Input: part model. Units: mm. Frame: model coordinates. Face numbers are marked on the shaded views. A direction names the side the tool comes from. Coordinates: 2 decimals unless noted, no trailing zeros. Loops run counter-clockwise (first coordinate to the right, second up) from the corner with the lowest first, then second, coordinate; pieces in that order, holes last. Notation, with made-up numbers: (-21, 19.5) - (-2, 19.5) arc R25 cw to (-2, 52.5) - close; hole circle Ø9 at (6.5, 55.25). An arc over 180 degrees is marked (long way). Use a Markdown table: item, result. Add a question column.
1. Section query B-B on z = 3.25. Return the cut outline in (x, y).
2. Draft query along X for the marked faces 4, 5 and 6. Return one class per face: released by +X, released by -X, zero draft, split by the parting line, or undercut.
3. Contact query for flat-ended pins moving along their axis: P1, Ø8, axis at y = -5.5, z = 8, coming from the +X side; P2, Ø1.9, axis at y = 27.5, z = -3.5, coming from the +X side; P3, Ø3.5, axis at y = 29.5, z = 4.5, coming from the -X side. Output: stop coordinate, or through.
4. Section query A-A on z = 7.5. Return the cut outline in (x, y).
5. Ray query, L1, parallel to Y at x = -4.5, z = 9; L2, parallel to X at y = -29, z = 1; L3, parallel to Z at x = 4, y = 5. Return the intervals inside material, ascending. Write a range as [from, to].
6. Section query C-C on y = -16. Return the cut outline in (x, z), then the cut area to 3 significant figures.
7. Section query D-D on x = 9.5. Return the cut outline in (y, z).
8. Access query for the marked faces 1, 2 and 3. Directions: +Z, -Z, +X, -X, +Y, -Y. A direction counts if a zero-diameter tool reaches every point of the face in a straight line with its end or side. Return the directions, or none.
```python
from build123d import *

# Parameters (mm, degrees)
F0_R           = 2.9845
F1_DEPTH       = 14.732
F2_W           = 7.293083705
F2_H           = 0.6463081809
F3_DEPTH       = 25.4
F4_R           = 25.4
F5_DEPTH       = 6.35
F7_DEPTH       = 6.35
F8_W           = 12.7
F8_H           = 6.858
F9_DEPTH       = 11.938
F11_DEPTH      = 25.4
F13_DEPTH      = 25.4
F14_W          = 5.7489185128
F14_H          = 1.582127763
F15_DEPTH      = 2.667
F17_R          = 3.0649258181
F18_DEPTH      = 5.08
F18_TAPER      = -3
F18_DEPTH_BACK = 2.54
F18_TAPER_BACK = 3


with BuildPart() as f1:
    # F0 (on Top) → F1 (new body)
    with BuildSketch(Plane.XY):
        Circle(F0_R)
    extrude(amount=F1_DEPTH)

    # F2 (on Top) → F3 (cut)
    with BuildSketch(Plane.XY):
        with Locations((-0.53606648, 0)):
            Rectangle(F2_W, F2_H)
    extrude(amount=F3_DEPTH, mode=Mode.SUBTRACT)



with BuildPart() as f5:
    # F4 (on Top) → F5 (new body)
    with BuildSketch(Plane.XY):
        Circle(F4_R)
    extrude(amount=-F5_DEPTH)


with BuildPart() as f7:
    # F6 (on Top) → F7 (new body)
    with BuildSketch(Plane.XY):
        Polygon((6.35, 33.02), (0, 33.02), (-6.35, 33.02), (-6.35, -33.02), (6.35, -33.02), align=None)
    extrude(amount=-F7_DEPTH)

    # F8 (on Top) → F9 (join)
    with BuildSketch(Plane.XY):
        with Locations((-0.1506691359, 29.6887743422)):
            Rectangle(F8_W, F8_H)
        with Locations((-0.1506691359, -29.5306027732)):
            Rectangle(F8_W, F8_H)
    extrude(amount=F9_DEPTH)

    # F10 (on Top) → F11 (cut)
    with BuildSketch(Plane.XY):
        Polygon((4.8673646525, -31.7627712542), (4.8673646525, -29.4287092984), (4.8673646525, -27.4035874754), (-1.8467506161, -27.4035874754), (-5.2787689492, -27.4035874754), (-5.2787689492, -29.4508635998), (-5.2787689492, -31.7627712542), align=None)
    extrude(amount=F11_DEPTH, mode=Mode.SUBTRACT)

    # F12 (on Top) → F13 (cut)
    with BuildSketch(Plane.XY):
        Polygon((-5.2687884308, 27.4780225009), (-1.7242872855, 27.4780225009), (4.8994985409, 27.4780225009), (4.8994985409, 29.8927128315), (4.8994985409, 31.842187047), (-0.8160090074, 31.842187047), (-5.2687884308, 31.842187047), (-5.2687884308, 29.5382626355), align=None)
    extrude(amount=F13_DEPTH, mode=Mode.SUBTRACT)


with BuildPart() as f15:
    # F14 (on face) → F15 (new body)
    with BuildSketch(Plane.XY):
        with Locations((-0.009511481, 0.0064342166)):
            Rectangle(F14_W, F14_H)
    extrude(amount=F15_DEPTH)


with BuildPart() as f1_1:
    add(f1.part)

    add(f5.part)  # F18 merges F5

    add(f7.part)  # F18 merges F7

    add(f15.part)  # F18 merges F15
    # F17 (on offset) → F18 (join, two sides)
    with BuildSketch(Plane.XY.offset(2.032)) as f18_sk:
        with Locations((-0.0702725374, 0)):
            Circle(F17_R)
    extrude(amount=-F18_DEPTH, taper=F18_TAPER)
    extrude(f18_sk.sketch, amount=F18_DEPTH_BACK, taper=F18_TAPER_BACK)


solid = f1_1.part
```
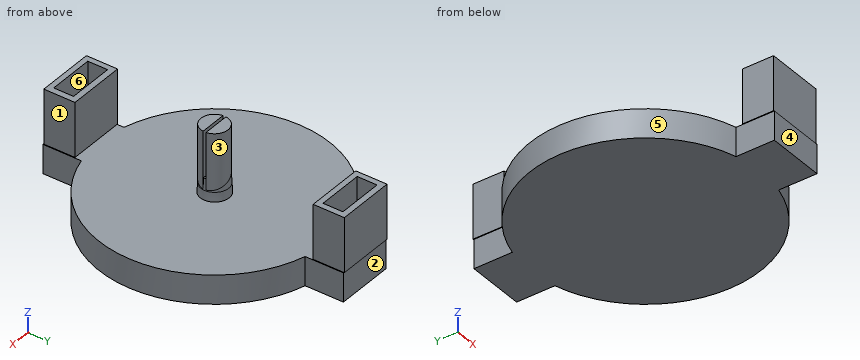
Resolved:
| question | item | result |
|---|---|---|
| 1 | outline | (-6.5, -32.96) - (6.2, -32.96) - (6.2, -26.1) - (-6.5, -26.1) - close; (-6.5, 26.26) - (6.2, 26.26) - (6.2, 33.12) - (-6.5, 33.12) - close; (0.67, -2.91) arc R2.98 ccw to (2.97, -0.32) - (2.91, -0.32) arc R3 ccw to (2.91, 0.32) - (2.97, 0.32) arc R2.98 ccw to (0.67, 2.91) arc R3 ccw (long way) to start; hole (-5.28, -31.76) - (4.87, -31.76) - (4.87, -27.4) - (-5.28, -27.4) - close; hole (-5.27, 27.48) - (4.9, 27.48) - (4.9, 31.84) - (-5.27, 31.84) - close |
| 2 | face 4 | zero draft |
| 2 | face 5 | released by -X |
| 2 | face 6 | undercut |
| 3 | P1 | x = 2.58 |
| 3 | P2 | x = 6.35 |
| 3 | P3 | x = -6.5 |
| 4 | outline | (-6.5, -32.96) - (6.2, -32.96) - (6.2, -26.1) - (-6.5, -26.1) - close; (-6.5, 26.26) - (6.2, 26.26) - (6.2, 33.12) - (-6.5, 33.12) - close; (-2.97, -0.32) arc R2.98 ccw to (2.97, -0.32) - close; (-2.97, 0.32) - (2.97, 0.32) arc R2.98 ccw to start; hole (-5.28, -31.76) - (4.87, -31.76) - (4.87, -27.4) - (-5.28, -27.4) - close; hole (-5.27, 27.48) - (4.9, 27.48) - (4.9, 31.84) - (-5.27, 31.84) - close |
| 5 | L1 | [-32.96, -31.76], [-27.4, -26.1], [26.26, 27.48], [31.84, 33.12] |
| 5 | L2 | [-6.5, -5.28], [4.87, 6.2] |
| 5 | L3 | [-6.35, 0] |
| 6 | outline | (-19.73, -6.35) - (19.73, -6.35) - (19.73, 0) - (-19.73, 0) - close |
| 6 | area | 251 mm² |
| 7 | outline | (-23.56, -6.35) - (23.56, -6.35) - (23.56, 0) - (-23.56, 0) - close |
| 8 | face 1 | +Z, +X, +Y, -Y |
| 8 | face 2 | -Z, +X, -X, +Y |
| 8 | face 3 | +Z |
